from build123d import *

# Parameters (mm, degrees)
SKETCH1_W           = 152.4
SKETCH1_H           = 114.3
BOSS_EXTRUDE1_DEPTH = 152.4
FILLET1_R           = 12.7


with BuildPart() as part:
    # Sketch1 → Boss-Extrude1 (new body)
    with BuildSketch(Plane(origin=(0, 0, 0), x_dir=(1, 0, 0), z_dir=(0, 1, 0))):
        Rectangle(SKETCH1_W, SKETCH1_H)
        with BuildLine():
            Line((-19.05, 31.75), (19.05, 31.75))
            ThreePointArc((19.05, 31.75), (50.8, 0), (19.05, -31.75))
            Line((19.05, -31.75), (-19.05, -31.75))
            ThreePointArc((-19.05, -31.75), (-50.8, 0), (-19.05, 31.75))
        make_face(mode=Mode.SUBTRACT)
    extrude(amount=BOSS_EXTRUDE1_DEPTH)

    # Fillet1
    fillet1_edges = [part.edges().sort_by_distance(p)[0] for p in [
        (-76.2, 152.4, 0),
        (0, 152.4, 57.15),
        (76.2, 152.4, 0),
        (0, 0, 57.15),
        (-76.2, 0, 0),
        (0, 0, -57.15),
        (76.2, 0, 0),
        (76.2, 76.2, 57.15),
        (-76.2, 76.2, 57.15),
        (-76.2, 76.2, -57.15),
        (76.2, 76.2, -57.15),
        (0, 152.4, -57.15),
    ]]
    fillet(fillet1_edges, radius=FILLET1_R)


solid = part.part
Can you work these out from the model? Positions are in its coordinate system, mm. A direction names the side the tool comes from. Round coordinates to 2 decimals unless told otherwise and drop trailing zeros. Write each loop counter-clockwise with the first axis right and the second up, starting at its lowest first coordinate (ties: lowest second). Pieces come first, ordered by that corner, then holes. Notation, with made-up numbers: M -36,48.5 L -17,48.5 A20 cw -17,53.5 Z; hole C 21.5,-9.75 d11. An arc over 180 degrees is marked long. Use CSV: the item, a comma, the result in double quotes.
(1) Imagine slicing it at A-A (z = 0). Write out the boundary of the cut face in (x, y).
Check values:
outline,"M -76.2,12.7 A12.7 ccw -63.5,0 L -50.8,0 L -50.8,152.4 L -63.5,152.4 A12.7 ccw -76.2,139.7 Z; M 50.8,0 L 63.5,0 A12.7 ccw 76.2,12.7 L 76.2,139.7 A12.7 ccw 63.5,152.4 L 50.8,152.4 Z"
(2) Imagine slicing it at C-C (y = 77.5). Write out the boundary of the cut face in (x, z).
Check values:
outline,"M -76.2,-44.45 A12.7 ccw -63.5,-57.15 L 63.5,-57.15 A12.7 ccw 76.2,-44.45 L 76.2,44.45 A12.7 ccw 63.5,57.15 L -63.5,57.15 A12.7 ccw -76.2,44.45 Z; hole M -19.05,-31.75 L 19.05,-31.75 A31.75 ccw 19.05,31.75 L -19.05,31.75 A31.75 ccw Z"
(3) We'd pull the mould along X, two halves only. Please class faces 3 (the cylindrical face through (72.38, 77.09, 53.53)), 4 (the flat face through (-1, 75, 57.15)), 5 (the cylindrical face through (-72.58, 3.82, -0.62)), 6 (the cylindrical face through (50.792, 75.133, -0.698)): +X half, -X half, draft (parallel to the pull), parting line (faces both ways), or undercut.
Check values:
face 3,"+X half"
face 4,"draft"
face 5,"-X half"
face 6,"undercut"
(4) Imagine slicing it at D-D (z = -49.5). Write out the boundary of the cut face in (x, y).
Check values:
outline,"M -75.15,12.7 A11.65 ccw -63.5,1.05 L 63.5,1.05 A11.65 ccw 75.15,12.7 L 75.15,139.7 A11.65 ccw 63.5,151.35 L -63.5,151.35 A11.65 ccw -75.15,139.7 Z"
(5) Imagine slicing it at B-B (x = -7). Write out the boundary of the cut face in (y, z), plus the area to 3 significant figures.
Check values:
outline,"M 0,-44.45 A12.7 ccw 12.7,-57.15 L 139.7,-57.15 A12.7 ccw 152.4,-44.45 L 152.4,-31.75 L 0,-31.75 Z; M 0,31.75 L 152.4,31.75 L 152.4,44.45 A12.7 ccw 139.7,57.15 L 12.7,57.15 A12.7 ccw 0,44.45 Z"
area,"7,600 mm^2"
(6) I need wall thicknesses on line 1 along Z through (x, y) = (-15, 118); line 2 along Z through (x, y) = (-41.5, 89); line 3 along X through (y, z) = (113.5, 23.5). Which ranges of each line are inside material? Lowest first, please.
Check values:
line 1,"-57.15 to -31.75, 31.75 to 57.15"
line 2,"-57.15 to -22.45, 22.45 to 57.15"
line 3,"-76.2 to -40.4, 40.4 to 76.2"
(7) On a 3-axis mill with a long thin cutter (end or side, diameter ignored), from which of +Z, -Z, +X, -X, +Y, -Y can I reach the whole of each face in a straight line? I mean faces 1 (the flat face through (76.2, 75, 1)), 2 (the cylindrical face through (-50.792, 75.133, 0.698)). Say none if no direction works.
Check values:
face 1,"+Z, -Z, +X, +Y, -Y"
face 2,"+Y, -Y"
